For this review, use the dimensioned drawing (mm, ordinates from the lowest corner) and the shaded views. Coordinates: 2 decimals unless noted, no trailing zeros. Order: outer loops, then holes, each group sorted by start corner. A loop starts at its lowest first (then second) coordinate and runs counter-clockwise, first axis right, second up. Notation, with made-up numbers: (76, -33.5) -> (134, -33.5) arc R25 ccw to (134, -8.5) -> close; hole circle Ø1 at (81.25, 20). An arc over 180 degrees is marked (long way). Use one line per item in the form item = value. Start each with the question number.
(1) Take a section at C-C (x = 150). State the section outline as (y, z) points.
(2) Take a section at B-B (z = 78.25). State the section outline as (x, y) points, then the cut area to 3 significant figures.
(3) Take a section at A-A (y = 2.4). State the section outline as (x, z) points, then the cut area to 3 significant figures.
(4) Wall thickness on line 1 along X through (y, z) = (2.1, 290); line 2 along Z through (x, y) = (150, 0.9): over which ranges is each line inside the solid? List them lowest first.
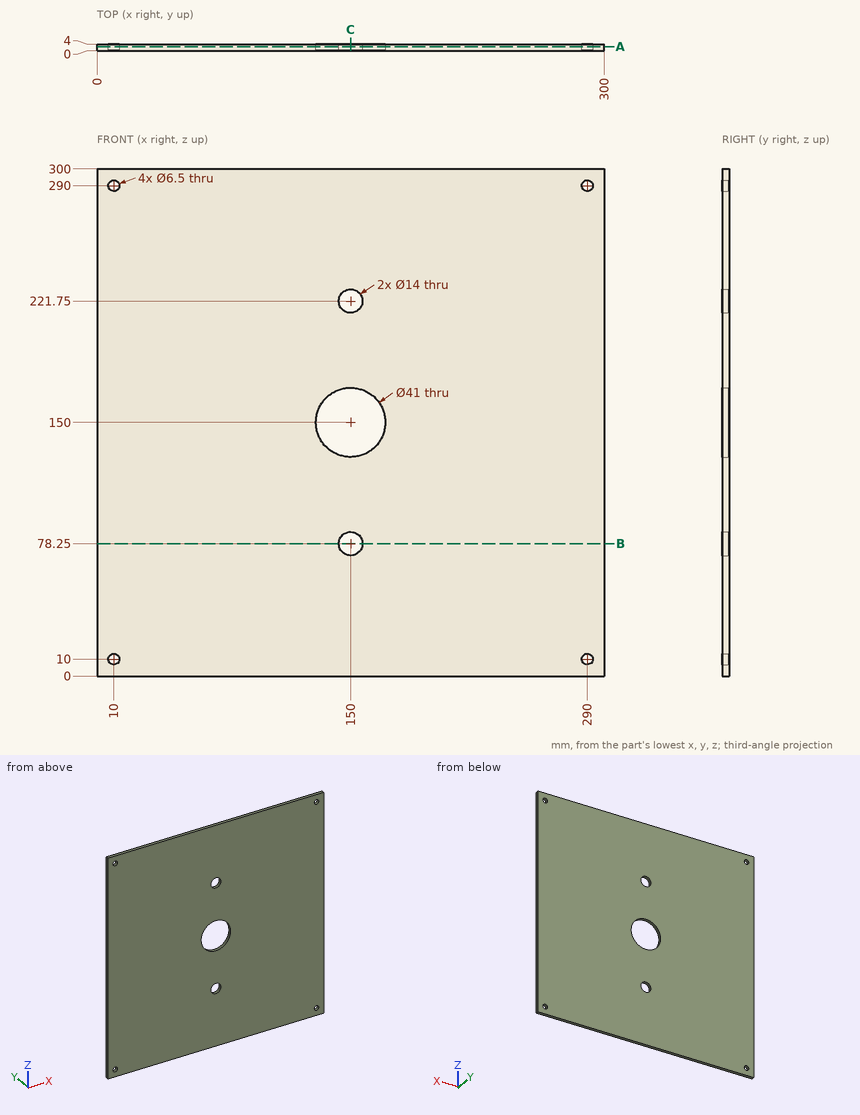
Findings:
q1.outline = (0, 0) -> (4, 0) -> (4, 71.25) -> (0, 71.25) -> close; (0, 85.25) -> (4, 85.25) -> (4, 129.5) -> (0, 129.5) -> close; (0, 170.5) -> (4, 170.5) -> (4, 214.75) -> (0, 214.75) -> close; (0, 228.75) -> (4, 228.75) -> (4, 300) -> (0, 300) -> close
q2.outline = (0, 0) -> (143, 0) -> (143, 4) -> (0, 4) -> close; (157, 0) -> (300, 0) -> (300, 4) -> (157, 4) -> close
q2.area = 1,140 mm²
q3.outline = (0, 0) -> (300, 0) -> (300, 300) -> (0, 300) -> close; hole circle Ø6.5 at (10, 10); hole circle Ø6.5 at (10, 290); hole circle Ø41 at (150, 150); hole circle Ø14 at (150, 78.25); hole circle Ø14 at (150, 221.75); hole circle Ø6.5 at (290, 10); hole circle Ø6.5 at (290, 290)
q3.area = 88,200 mm²
q4.line_1 = 0 to 6.75, 13.25 to 286.75, 293.25 to 300
q4.line_2 = 0 to 71.25, 85.25 to 129.5, 170.5 to 214.75, 228.75 to 300
